Geometry: final body of the model. Coordinates: model frame, mm. Face numbers are marked on the shaded views. A direction names the side the tool comes from. Coordinates: 2 decimals unless noted, no trailing zeros. Order: outer loops, then holes, each group sorted by start corner. A loop starts at its lowest first (then second) coordinate and runs counter-clockwise, first axis right, second up. Notation, with made-up numbers: (30.25, 17) - (76.25, 17) arc R25 ccw to (76.25, 49) - close; hole circle Ø3 at (7, 88.5). An arc over 180 degrees is marked (long way). Use a Markdown table: item, result. Add a question column.
```python
from build123d import *

# Parameters (mm, degrees)
SKETCH1_W               = 190
SKETCH1_H               = 120
BOSS_EXTRUDE1_DEPTH     = 260
FILLET1_R               = 42.5
SKETCH2_W               = 13
SKETCH2_H               = 22
BOSS_EXTRUDE2_DEPTH     = 8
CUT_EXTRUDE5_DEPTH      = 32
CUT_EXTRUDE6_DEPTH      = 32
BOSS_EXTRUDE3_DEPTH     = 2
SKETCH10_R              = 33
CUT_EXTRUDE7_DEPTH      = 2.5
MIRROR3_COPY_1_SKETCH_R = 33
MIRROR3_COPY_1_DEPTH    = 2.5
SKETCH11_W              = 98.911006982
SKETCH11_H              = 120
BOSS_EXTRUDE4_DEPTH     = 60
FILLET2_R               = 20
CUT_EXTRUDE8_REACH      = 465.953


with BuildPart() as part:
    # Sketch1 → Boss-Extrude1 (new body)
    with BuildSketch(Plane.XY):
        with Locations((40.07989685, -36.299360248)):
            Rectangle(SKETCH1_W, SKETCH1_H)
    extrude(amount=-BOSS_EXTRUDE1_DEPTH)

    # Fillet1
    fillet1_edges = [part.edges().sort_by_distance(p)[0] for p in [
        (-54.92010315, 23.700639752, -130),
        (135.07989685, 23.700639752, -130),
        (135.07989685, -96.299360248, -130),
        (-54.92010315, -96.299360248, -130),
    ]]
    fillet(fillet1_edges, radius=FILLET1_R)

    # Sketch2 → Boss-Extrude2 (add)
    with BuildSketch(Plane(origin=(0, 23.700639752, 0), x_dir=(1, 0, 0), z_dir=(0, 1, 0))):
        with Locations((-0.67010315, 243)):
            Rectangle(SKETCH2_W, SKETCH2_H)
        with Locations((80.82989685, 243)):
            Rectangle(SKETCH2_W, SKETCH2_H)
        with Locations((-0.67010315, 17)):
            Rectangle(SKETCH2_W, SKETCH2_H)
        with Locations((80.82989685, 17)):
            Rectangle(SKETCH2_W, SKETCH2_H)
    extrude(amount=BOSS_EXTRUDE2_DEPTH)

    # Sketch5 → Cut-Extrude5 (cut)
    with BuildSketch(Plane(origin=(0, 0, -254), x_dir=(-1, 0, 0), z_dir=(0, 0, -1))):
        Polygon((-87.32989685, 23.700639752), (-81.32989685, 31.700639752), (-87.32989685, 31.700639752), align=None)
    cut_extrude5 = extrude(amount=-CUT_EXTRUDE5_DEPTH, mode=Mode.SUBTRACT)

    # Sketch7 → Cut-Extrude6 (cut)
    with BuildSketch(Plane(origin=(0, 0, -254), x_dir=(-1, 0, 0), z_dir=(0, 0, -1))):
        Polygon((1.17010315, 31.700639752), (7.17010315, 23.700639752), (7.17010315, 31.700639752), align=None)
    cut_extrude6 = extrude(amount=-CUT_EXTRUDE6_DEPTH, mode=Mode.SUBTRACT)

    # Mirror1: Cut-Extrude5, Cut-Extrude6 across plane
    add(cut_extrude5.mirror(Plane.XY.offset(-130)), mode=Mode.SUBTRACT)
    add(cut_extrude6.mirror(Plane.XY.offset(-130)), mode=Mode.SUBTRACT)

    # Sketch9 → Boss-Extrude3 (add)
    with BuildSketch(Plane(origin=(0, 23.700639752, 0), x_dir=(1, 0, 0), z_dir=(0, 1, 0))):
        with BuildLine():
            ThreePointArc((13.944025684, 274.437502336), (11.227457344, 267.446426584), (10.32989685, 260))
            Line((10.32989685, 260), (10.32989685, 225))
            Line((10.32989685, 225), (20.57989685, 225))
            Line((20.57989685, 225), (61.829871341, 225))
            Line((61.829871341, 225), (70.32989685, 225))
            Line((70.32989685, 225), (70.32989685, 260))
            ThreePointArc((70.32989685, 260), (69.808755544, 265.731054618), (68.202935744, 271.257167))
            ThreePointArc((68.202935744, 271.257167), (58.544976128, 302.436051532), (60.82989685, 334.996428708))
            Line((60.82989685, 334.996428708), (60.82989685, 364.996428708))
            Line((60.82989685, 364.996428708), (19.82989685, 364.996428708))
            Line((19.82989685, 364.996428708), (19.82989685, 334.996428708))
            ThreePointArc((19.82989685, 334.996428708), (22.342438119, 304.186734294), (13.944025684, 274.437502336))
        make_face()
    boss_extrude3 = extrude(amount=-BOSS_EXTRUDE3_DEPTH)

    # Sketch10 → Cut-Extrude7 (cut, symmetric)
    with BuildSketch(Plane(origin=(0, 0, -260), x_dir=(-1, 0, 0), z_dir=(0, 0, -1))):
        with Locations((-85.07989685, -36.299360248)):
            Circle(SKETCH10_R)
    cut_extrude7 = extrude(amount=CUT_EXTRUDE7_DEPTH, both=True, mode=Mode.SUBTRACT)

    # Mirror2: Cut-Extrude7 across plane
    add(cut_extrude7.mirror(Plane(origin=(40.07989685, 0, 0), x_dir=(0, 0, 1), z_dir=(1, 0, 0))), mode=Mode.SUBTRACT)

    # Mirror3: Cut-Extrude7 across plane
    add(cut_extrude7.mirror(Plane.XY.offset(-130)), mode=Mode.SUBTRACT)

    # Mirror3 copy 1 sketch → Mirror3 copy 1 (cut, symmetric)
    with BuildSketch(Plane(origin=(80.1597937, 0, 0), x_dir=(1, 0, 0), z_dir=(0, 0, 1))):
        with Locations((-85.07989685, -36.299360248)):
            Circle(MIRROR3_COPY_1_SKETCH_R)
    extrude(amount=MIRROR3_COPY_1_DEPTH, both=True, mode=Mode.SUBTRACT)

    # Mirror4: Boss-Extrude3 across plane
    add(boss_extrude3.mirror(Plane.ZX.offset(-36.299360248)))

    # Sketch11 → Boss-Extrude4 (add)
    with BuildSketch(Plane(origin=(0, 0, -364.996428708), x_dir=(-1, 0, 0), z_dir=(0, 0, -1))):
        with Locations((-38.121760163, -36.299360248)):
            Rectangle(SKETCH11_W, SKETCH11_H)
    extrude(amount=BOSS_EXTRUDE4_DEPTH)

    # Fillet2
    fillet2_edges = [part.edges().sort_by_distance(p)[0] for p in [
        (87.577263654, 23.700639752, -394.996428708),
        (87.577263654, -96.299360248, -394.996428708),
        (-11.333743328, -96.299360248, -394.996428708),
        (-11.333743328, 23.700639752, -394.996428708),
        (87.577263654, -36.299360248, -424.996428708),
        (38.121760163, -96.299360248, -424.996428708),
        (-11.333743328, -36.299360248, -424.996428708),
        (38.121760163, 23.700639752, -424.996428708),
    ]]
    fillet(fillet2_edges, radius=FILLET2_R)

    # Sketch12 → Cut-Extrude8 (cut, up to next)
    with BuildSketch(Plane.XZ.offset(96.299360248), mode=Mode.PRIVATE) as cut_extrude8_sk1:
        with BuildLine():
            Line((-11.333743328, -384.996428708), (-11.333743328, -364.996428708))
            Line((-11.333743328, -364.996428708), (19.82989685, -364.996428708))
            add(Edge.make_bspline(
                [(-11.333743328, -384.996428708), (15.244679544, -393.728247891), (19.82989685, -364.996428708)],
                knots=[0, 0, 0, 1, 1, 1], degree=2))
        make_face()
    cut_extrude8_tool1 = extrude(cut_extrude8_sk1.sketch, amount=-CUT_EXTRUDE8_REACH, mode=Mode.PRIVATE) & part.part
    cut_extrude8 = cut_extrude8_tool1.solids().sort_by_distance((2.471753, -96.29936, -374.935763))[0]
    add(cut_extrude8, mode=Mode.SUBTRACT)

    # Mirror5: Cut-Extrude8 across plane
    add(cut_extrude8.mirror(Plane(origin=(40.07989685, 0, 0), x_dir=(0, 0, 1), z_dir=(1, 0, 0))), mode=Mode.SUBTRACT)


solid = part.part
```
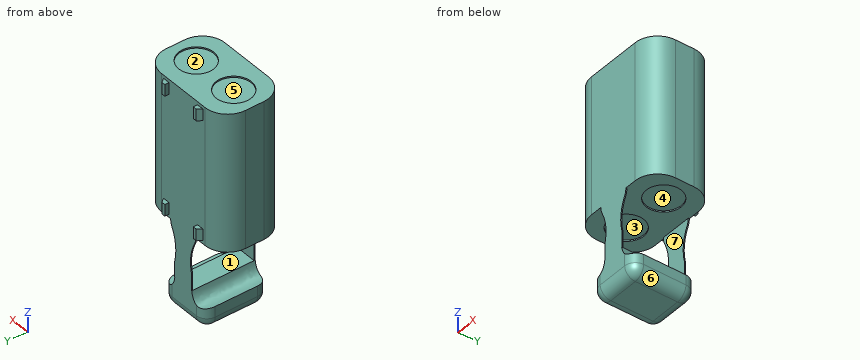
1) Line query: line 1 (Z direction, x = 54, y = -13.5); line 2 (Z direction, x = 122, y = -65); line 3 (Y direction, x = 79.5, z = -46). Output: solid intervals per line, ascending. Write a range as from..to.
2) Section query C-C (z = -397.5). Return the cut outline in (x, y).
3) Section query D-D (x = 110.5). Return the cut outline in (y, z), and give its area (3 significant figures).
4) First-contact query: pin 1 (4 mm diameter, centred on x = 50.5, y = -42, fed in from +Z); pin 2 (10 mm diameter, centred on y = -43.5, z = -396.5, fed in from -X); pin 3 (1 mm diameter, centred on y = -95.5, z = -347.5, fed in from -X); pin 4 (18 mm diameter, centred on x = 43.5, z = -311, fed in from +Y). Flat tips, straight axial feed; report the tip coordinate or a pass-through.
5) Section query A-A (z = -266). Return the cut outline in (x, y), and give its area (3 significant figures).
6) Draft query along Z for the marked faces 4, 5, 6 and 7. Return one class per face: released by +Z, released by -Z, zero draft, split by the parting line, or undercut.
7) Access query for the marked faces 1, 2 and 3. Directions: +Z, -Z, +X, -X, +Y, -Y. A direction counts if a zero-diameter tool reaches every point of the face in a straight line with its end or side. Return the directions, or none.
8) Section query B-B (x = 38). Return the cut outline in (y, z), and give its area (3 significant figures).
From the geometry:
| question | item | result |
|---|---|---|
| 1 | line 1 | z = -425..-365, -260..0 |
| 1 | line 2 | z = -260..0 |
| 1 | line 3 | y = -96.3..23.7 |
| 2 | outline | (-11.33, -76.3) arc R20 ccw to (8.67, -96.3) - (67.58, -96.3) arc R20 ccw to (87.58, -76.3) - (87.58, 3.7) arc R20 ccw to (67.58, 23.7) - (8.67, 23.7) arc R20 ccw to (-11.33, 3.7) - close |
| 3 | outline | (-92.34, -260) - (-57.34, -260) - (-57.34, -257.5) - (-15.26, -257.5) - (-15.26, -260) - (19.74, -260) - (19.74, 0) - (-15.26, 0) - (-15.26, -2.5) - (-57.34, -2.5) - (-57.34, 0) - (-92.34, 0) - close |
| 3 | area | 28,900 mm^2 |
| 4 | pin 1 | stops at z = 0 |
| 4 | pin 2 | stops at x = -11.33 |
| 4 | pin 3 | stops at x = 19.83 |
| 4 | pin 4 | stops at y = 23.7 |
| 5 | outline | (10.9, -96.3) - (69.76, -96.3) - (69.76, -94.3) - (10.9, -94.3) - close; (10.9, 21.7) - (69.76, 21.7) - (69.76, 23.7) - (10.9, 23.7) - close |
| 5 | area | 235 mm^2 |
| 6 | face 4 | undercut |
| 6 | face 5 | released by +Z |
| 6 | face 6 | released by -Z |
| 6 | face 7 | undercut |
| 7 | face 1 | +X, -X |
| 7 | face 2 | +Z |
| 7 | face 3 | none |
| 8 | outline | (-96.3, -405) arc R20 ccw to (-76.3, -425) - (3.7, -425) arc R20 ccw to (23.7, -405) - (23.7, 0) - (-96.3, 0) - close; hole (-94.3, -365) - (21.7, -365) - (21.7, -260) - (-94.3, -260) - close |
| 8 | area | 38,600 mm^2 |
